from build123d import *

# Parameters (mm, degrees)
F0_R     = 1.55
F0_W     = 8
F0_H     = 7
F0_R_2   = 0.75
F1_DEPTH = 28
F2_DEPTH = 27
F3_R     = 0.5
F4_R     = 0.5


with BuildPart() as f1:
    # F0 (on Front) → F1 (new body)
    with BuildSketch(Plane.XZ):
        with BuildLine():
            ThreePointArc((15, -4), (19, 0), (15, 4))
            Line((15, 4), (0, 4))
            Line((0, 4), (-15, 4))
            ThreePointArc((-15, 4), (-19, 0), (-15, -4))
            Line((-15, -4), (-12, -4))
            Line((-12, -4), (-12, -5))
            Line((-12, -5), (-12, -5.5))
            Line((-12, -5.5), (0, -5.5))
            Line((0, -5.5), (12, -5.5))
            Line((12, -5.5), (12, -5))
            Line((12, -5), (12, -4))
            Line((12, -4), (15, -4))
        make_face()
        with Locations((-15, 0)):
            Circle(F0_R, mode=Mode.SUBTRACT)
        with Locations((-5.906985, -0.57222)):
            Rectangle(F0_W, F0_H, mode=Mode.SUBTRACT)
        with Locations((5.906985, -0.57222)):
            Rectangle(F0_W, F0_H, mode=Mode.SUBTRACT)
        with Locations((15, 0)):
            Circle(F0_R, mode=Mode.SUBTRACT)
        with Locations((5.906985, -0.57222)):
            Rectangle(F0_W, F0_H)
        with Locations((5.906985, -0.57222)):
            Circle(F0_R_2, mode=Mode.SUBTRACT)
        with Locations((-5.906985, -0.57222)):
            Rectangle(F0_W, F0_H)
        with Locations((-5.906985, -0.57222)):
            Circle(F0_R_2, mode=Mode.SUBTRACT)
    extrude(amount=F1_DEPTH)

    # F0 (on Front) → F2 (cut)
    with BuildSketch(Plane.XZ):
        with Locations((5.906985, -0.57222)):
            Rectangle(F0_W, F0_H)
        with Locations((5.906985, -0.57222)):
            Circle(F0_R_2, mode=Mode.SUBTRACT)
        with Locations((-5.906985, -0.57222)):
            Rectangle(F0_W, F0_H)
        with Locations((-5.906985, -0.57222)):
            Circle(F0_R_2, mode=Mode.SUBTRACT)
    extrude(amount=F2_DEPTH, mode=Mode.SUBTRACT)

    # F3
    f3_edges = [f1.edges().sort_by_distance(p)[0] for p in [
        (0, 0, 4),
        (-13.5, 0, -4),
        (0, 0, -5.5),
        (-12, 0, -4.75),
        (12, 0, -4.75),
        (13.5, 0, -4),
        (19, 0, 0),
        (-19, 0, 0),
    ]]
    fillet(f3_edges, radius=F3_R)

    # F4
    f4_edges = [f1.edges().sort_by_distance(p)[0] for p in [
        (0, -28, 4),
        (-19, -28, 0),
        (-13.5, -28, -4),
        (-12, -28, -4.75),
        (0, -28, -5.5),
        (12, -28, -4.75),
        (13.5, -28, -4),
        (19, -28, 0),
    ]]
    fillet(f4_edges, radius=F4_R)


solid = f1.part
Check sheet for the modelled part. Datum: model origin and axes. Units: mm. A direction names the side the tool comes from. Give positions to 0.01 mm unless a question says otherwise; leave off trailing zeros. Write each loop counter-clockwise with the first axis right and the second up, starting at its lowest first coordinate (ties: lowest second). Pieces come first, ordered by that corner, then holes. Notation, with made-up numbers: (85, 74) -> (90, 74) arc R13 cw to (90, 97) -> close; hole circle Ø11 at (79.25, -30.75). An arc over 180 degrees is marked (long way). One line per item, written item: value. Start each with the question number.
Item 1: Draft check along Z on faces 5 (the flat face through (13, -14, -4)), 6 (the flat face through (-6, -13, -4.072)), 7 (the flat face through (0, -28, -1)). Enter one of: +Z half, -Z half, draft (parallel to the pull), parting line (faces both ways), or undercut.
Item 2: Section check B-B on x = 13. Record the cut outline in (y, z), then the cut area to 3 significant figures.
Item 3: Material ranges on probe 1 along Z at (x, y) = (9, -10); probe 2 along X at (y, z) = (-5.5, -0.25); probe 3 along Z at (x, y) = (15, -6.5), recorded low to high. Write a range as from..to.
Item 4: Tool access check on faces 1 (the flat face through (12, -14, -5)), 2 (the cylindrical face through (-19, -14, 0)), 3 (the flat face through (6, -13, -4.072)), 4 (the flat face through (-12, -14, -5)). Record the directions out of +Z, -Z, +X, -X, +Y, -Y that give a thin tool (end or side, any length) a straight path to the whole face; none if there is none.
Item 5: Gauge pin test, flat ends, axial feed: pin 1 (5.5 mm diameter, centred on x = -7, z = -0.5, fed in from +Y); pin 2 (2.5 mm diameter, centred on x = -14, y = -11.5, fed in from -Z); pin 3 (1.2 mm diameter, centred on y = -12.5, z = -5, fed in from +X). Record the tip position at first contact, or that the pin passes through.
Item 6: Section check C-C on x = -9.5. Record the cut outline in (y, z).
Item 7: Section check A-A on y = -15. Record the cut outline in (x, z).
Results list:
1. face 5: -Z half
1. face 6: undercut
1. face 7: draft
2. outline: (-28, -3.5) arc R0.5 ccw to (-27.5, -4) -> (-0.5, -4) arc R0.5 ccw to (0, -3.5) -> (0, 3.5) arc R0.5 ccw to (-0.5, 4) -> (-27.5, 4) arc R0.5 ccw to (-28, 3.5) -> close
2. area: 224 mm²
3. probe 1: -5.5..-4.07, 2.93..4
3. probe 2: -18.99..-16.53, -13.47..-9.91, -1.91..1.91, 9.91..13.47, 16.53..18.99
3. probe 3: -4..-1.55, 1.55..4
4. face 1: -Z, +X, +Y, -Y
4. face 2: -X, +Y, -Y
4. face 3: +Y
4. face 4: -Z, -X, +Y, -Y
5. pin 1: y = -27
5. pin 2: z = -4
5. pin 3: x = 12
6. outline: (-28, -5) arc R0.5 ccw to (-27.5, -5.5) -> (-0.5, -5.5) arc R0.5 ccw to (0, -5) -> (0, -4.07) -> (-27, -4.07) -> (-27, 2.93) -> (0, 2.93) -> (0, 3.5) arc R0.5 ccw to (-0.5, 4) -> (-27.5, 4) arc R0.5 ccw to (-28, 3.5) -> close
7. outline: (-15, -4) -> (-12, -4) -> (-12, -5.5) -> (12, -5.5) -> (12, -4) -> (15, -4) arc R4 ccw to (15, 4) -> (-15, 4) arc R4 ccw to start; hole circle Ø3.1 at (-15, 0); hole (-9.91, -4.07) -> (-1.91, -4.07) -> (-1.91, 2.93) -> (-9.91, 2.93) -> close; hole (1.91, -4.07) -> (9.91, -4.07) -> (9.91, 2.93) -> (1.91, 2.93) -> close; hole circle Ø3.1 at (15, 0)
